```python
from build123d import *

# Parameters (mm, degrees)
SKETCH1_R           = 6
BOSS_EXTRUDE1_DEPTH = 4
SKETCH2_R           = 4.5
BOSS_EXTRUDE2_DEPTH = 14
SKETCH3_W           = 5
SKETCH3_H           = 5
CUT_EXTRUDE1_DEPTH  = 4
SKETCH4_R           = 3
CUT_EXTRUDE2_DEPTH  = 10
BOSS_EXTRUDE3_START = 10
BOSS_EXTRUDE3_DEPTH = 10


with BuildPart() as part:
    # Sketch1 → Boss-Extrude1 (new body)
    with BuildSketch(Plane(origin=(0, 0, 0), x_dir=(1, 0, 0), z_dir=(0, 1, 0))):
        with Locations(Location((0, 0, 0), (0, 0, 270))):
            Circle(SKETCH1_R)
    extrude(amount=BOSS_EXTRUDE1_DEPTH)

    # Sketch2 → Boss-Extrude2 (add)
    with BuildSketch(Plane(origin=(0, 4, 0), x_dir=(1, 0, 0), z_dir=(0, 1, 0))):
        with Locations(Location((0, 0, 0), (0, 0, 270))):
            Circle(SKETCH2_R)
    extrude(amount=BOSS_EXTRUDE2_DEPTH)

    # Sketch3 → Cut-Extrude1 (cut)
    with BuildSketch(Plane(origin=(0, 0, 0), x_dir=(-1, 0, 0), z_dir=(0, -1, 0))):
        Rectangle(SKETCH3_W, SKETCH3_H)
    extrude(amount=-CUT_EXTRUDE1_DEPTH, mode=Mode.SUBTRACT)

    # Sketch4 → Cut-Extrude2 (cut)
    with BuildSketch(Plane(origin=(0, 18, 0), x_dir=(1, 0, 0), z_dir=(0, 1, 0))):
        with Locations(Location((0, 0, 0), (0, 0, 270))):
            Circle(SKETCH4_R)
    extrude(amount=-CUT_EXTRUDE2_DEPTH, mode=Mode.SUBTRACT)

    # Sketch5 → Boss-Extrude3 (add)
    with BuildSketch(Plane(origin=(0, 8, 0), x_dir=(1, 0, 0), z_dir=(0, 1, 0)).offset(BOSS_EXTRUDE3_START)):
        with BuildLine():
            Line((-1.65486069, -2.502286174), (-1.33961305, 2.684294484))
            ThreePointArc((-1.33961305, 2.684294484), (-2.994473739, 0.18200831), (-1.65486069, -2.502286174))
        make_face()
    extrude(amount=-BOSS_EXTRUDE3_DEPTH)


solid = part.part
```
Input: part model. Units: mm. Frame: model coordinates. A direction names the side the tool comes from. Give positions to 0.01 mm unless a question says otherwise; leave off trailing zeros. Order: outer loops, then holes, each group sorted by start corner. A loop starts at its lowest first (then second) coordinate and runs counter-clockwise, first axis right, second up. Notation, with made-up numbers: (-12, -3.5) - (16, -3.5) arc R34 cw to (16, 33.5) - close; hole circle Ø11 at (-24, -7.5). An arc over 180 degrees is marked (long way). Use a Markdown table: item, result.
(1) Access query for faces 4 (the flat face through (-1.5, 13.07, -0.05)), 5 (the flat face through (-2.5, 2, 0)), 6 (the flat face through (-2, 18, 0)). Directions: +Z, -Z, +X, -X, +Y, -Y. A direction counts if a zero-diameter tool reaches every point of the face in a straight line with its end or side. Return the directions, or none.
Computed values:
| item | result |
|---|---|
| face 4 | +Y |
| face 5 | -Y |
| face 6 | +Z, -Z, +X, -X, +Y |
(2) Draft query along Z for faces 1 (the cylindrical face through (1.802, 1.972, 5.723)), 2 (the flat face through (4.5, 4, -1.4)), 3 (the flat face through (2.5, 2, 0)). Return one class per face: released by +Z, released by -Z, zero draft, split by the parting line, or undercut.
Computed values:
| item | result |
|---|---|
| face 1 | split by the parting line |
| face 2 | zero draft |
| face 3 | undercut |
(3) Section query C-C (z = 0). Output: boundary loops of the cut face in (x, y), then the cut area to 3 significant figures.
Computed values:
| item | result |
|---|---|
| outline | (-6, 0) - (-2.5, 0) - (-2.5, 4) - (2.5, 4) - (2.5, 0) - (6, 0) - (6, 4) - (4.5, 4) - (4.5, 18) - (3, 18) - (3, 8) - (-1.5, 8) - (-1.5, 18) - (-4.5, 18) - (-4.5, 4) - (-6, 4) - close |
| area | 109 mm2 |
(4) Section query B-B (y = 17.25). Output: boundary loops of the cut face in (x, z), then the cut area to 3 significant figures.
Computed values:
| item | result |
|---|---|
| outline | circle Ø9 at (0, 0); hole (-1.65, 2.5) - (-1.34, -2.68) arc R3 ccw (long way) to start |
| area | 40.9 mm2 |
(5) Section query A-A (x = 0). Output: boundary loops of the cut face in (y, z), then the cut area to 3 significant figures.
Computed values:
| item | result |
|---|---|
| outline | (0, -6) - (4, -6) - (4, -4.5) - (18, -4.5) - (18, -3) - (8, -3) - (8, 3) - (18, 3) - (18, 4.5) - (4, 4.5) - (4, 6) - (0, 6) - (0, 2.5) - (4, 2.5) - (4, -2.5) - (0, -2.5) - close |
| area | 94.0 mm2 |
(6) Section query D-D (y = 5). Output: boundary loops of the cut face in (x, z), then the cut area to 3 significant figures.
Computed values:
| item | result |
|---|---|
| outline | circle Ø9 at (0, 0) |
| area | 63.6 mm2 |
(7) Pin query (flat end, axial travel): pin 1 (3 mm diameter, centred on y = 7, z = -5, fed in from +X); pin 2 (3 mm diameter, centred on x = -1, y = 8.5, fed in from +Z); pin 3 (1.5 mm diameter, centred on x = 1, z = 0, fed in from -Y). Return the tip coordinate at first contact, or that it passes through.
Computed values:
| item | result |
|---|---|
| pin 1 | stops at x = 2.83 |
| pin 2 | stops at z = 4.5 |
| pin 3 | stops at y = 4 |
(8) Line query: line 1 (Y direction, x = -3.5, z = -4.5); line 2 (X direction, y = 13.25, z = 0); line 3 (Z direction, x = 2.5, y = 15.25). Output: solid intervals per line, ascending. Write a range as from..to.
Computed values:
| item | result |
|---|---|
| line 1 | y = 0..4 |
| line 2 | x = -4.5..-1.5, 3..4.5 |
| line 3 | z = -3.74..-1.66, 1.66..3.74 |
